Could you check a few things on this drawing? It's one solid part, dimensions in mm from its lowest x, y, z. Give positions to 0.01 mm unless a question says otherwise; leave off trailing zeros. Order: outer loops, then holes, each group sorted by start corner. A loop starts at its lowest first (then second) coordinate and runs counter-clockwise, first axis right, second up. Notation, with made-up numbers: (-17, 43.25) - (2, 43.25) arc R20 cw to (2, 66.25) - close; hole circle Ø11 at (7, 9). An arc over 180 degrees is marked (long way). Return JSON: item names as keys, results as strings.
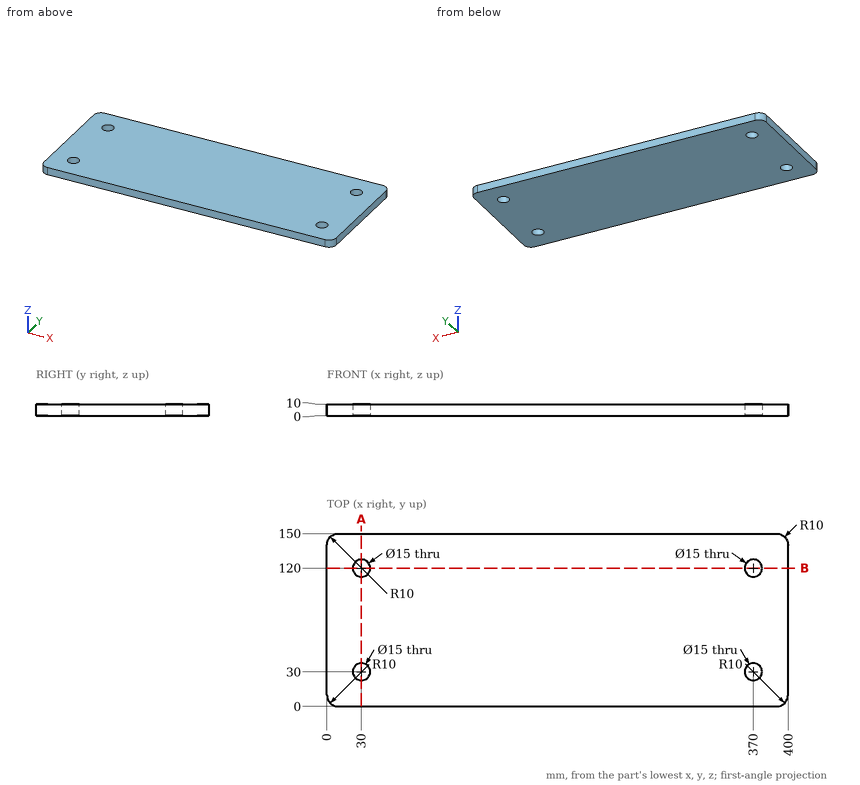
1. If I drill on L1, parallel to Y at x = 30, z = 5; L2, parallel to Y at x = 26, z = 7; L3, parallel to X at y = 33.5, z = 5, over which ranges is the centre line in solid material (lowest first)? Write a range as [from, to].
Checks:
{"L1": "[0, 22.5], [37.5, 112.5], [127.5, 150]", "L2": "[0, 23.66], [36.34, 113.66], [126.34, 150]", "L3": "[0, 23.37], [36.63, 363.37], [376.63, 400]"}
2. Suppose I cut it at A-A (x = 30). List the corners of the cut face in (y, z) for me.
Checks:
{"outline": "(0, 0) - (22.5, 0) - (22.5, 10) - (0, 10) - close; (37.5, 0) - (112.5, 0) - (112.5, 10) - (37.5, 10) - close; (127.5, 0) - (150, 0) - (150, 10) - (127.5, 10) - close"}
3. Suppose I cut it at B-B (y = 120). List the corners of the cut face in (x, z) for me.
Checks:
{"outline": "(0, 0) - (22.5, 0) - (22.5, 10) - (0, 10) - close; (37.5, 0) - (362.5, 0) - (362.5, 10) - (37.5, 10) - close; (377.5, 0) - (400, 0) - (400, 10) - (377.5, 10) - close"}
